Verification items for the finished model (mm, model axes). A direction names the side the tool comes from. Coordinates: 2 decimals unless noted, no trailing zeros. Order: outer loops, then holes, each group sorted by start corner. A loop starts at its lowest first (then second) coordinate and runs counter-clockwise, first axis right, second up. Notation, with made-up numbers: M 51,82 L 62,82 A17 cw 62,94 Z; hole C -3,-40 d4. An arc over 180 degrees is marked long. Answer as a JSON object with one key per item and string values. Group by question number.
(1) Cross-section at A-A (z = 15). Enter the section's corners in (x, y), plus the area to 3 significant figures.
(2) Access from +Z, -Z, +X, -X, +Y, -Y to the whole of each face (thin tool, end or side, straight path). Record for faces 5 (the face through (-12.5, 6, -1)), 6 (the face through (0, -5.5, 27)), 7 (the face through (-15.5, 5, 0)).
(3) Mould release check, pull along X, two halves, no side actions. Record for faces 1 (the face through (20, 11, -13)), 2 (the face through (-0.341, -15.496, 0.399)), 3 (the face through (16, 12.5, 0)), 4 (the face through (23.5, 11, 0)): released by +X, released by -X, zero draft, split by the parting line, or undercut.
(4) Gauge pin test, flat ends, axial feed: pin 1 Ø4 at (y, z) = (4.5, 4.5) entering from +X; pin 2 Ø6 at (x, z) = (10, -10) entering from +Y; pin 3 Ø1.5 at (y, z) = (0.5, 27.5) entering from -X; pin 4 Ø6.5 at (x, z) = (17.5, 11.5) entering from -Y. Record the tip position at first contact, or that the pin passes through.
(5) Cross-section at D-D (x = 10). Enter the section's corners in (y, z), plus the area to 3 significant figures.
(6) Cross-section at C-C (z = -19). Enter the section's corners in (x, y).
(7) Cross-section at B-B (x = -18). Enter the section's corners in (y, z), plus the area to 3 significant figures.
(8) Material ranges on line 1 (Z direction, x = -18, y = 11.95); line 2 (X direction, y = 0.25, z = -4); line 3 (Y direction, x = 0, z = 20), recorded low to high.
from build123d import *

# Parameters (mm, degrees)
SALIENTE_EXTRUIR1_DEPTH = 28.5
CROQUIS2_R              = 2
CORTAR_EXTRUIR1_DEPTH   = 5
SALIENTE_EXTRUIR2_DEPTH = 3
CROQUIS4_W              = 5
CROQUIS4_H              = 3
CROQUIS4_W_2            = 7
CROQUIS4_H_2            = 13
CORTAR_EXTRUIR3_DEPTH   = 3


with BuildPart() as part:
    # Croquis1 → Saliente-Extruir1 (new, symmetric)
    with BuildSketch(Plane.XY):
        with BuildLine():
            Line((-12.5, 0), (-12.5, 12.5))
            Line((-12.5, 12.5), (-23.5, 12.5))
            Line((-23.5, 12.5), (-23.5, 9.5))
            Line((-23.5, 9.5), (-15.5, 9.5))
            Line((-15.5, 9.5), (-15.5, 0))
            ThreePointArc((-15.5, 0), (0, -15.5), (15.5, 0))
            Line((15.5, 0), (15.5, 9.5))
            Line((15.5, 9.5), (23.5, 9.5))
            Line((23.5, 9.5), (23.5, 12.5))
            Line((23.5, 12.5), (12.5, 12.5))
            Line((12.5, 12.5), (12.5, 0))
            ThreePointArc((12.5, 0), (0, -12.5), (-12.5, 0))
        make_face()
    extrude(amount=SALIENTE_EXTRUIR1_DEPTH, both=True)

    # Croquis2 → Cortar-Extruir1 (cut)
    with BuildSketch(Plane.XZ.offset(-9.5)):
        with Locations((-18, 15)):
            Circle(CROQUIS2_R)
        with Locations((-18, -15)):
            Circle(CROQUIS2_R)
        with Locations((20, 15)):
            Circle(CROQUIS2_R)
        with Locations((20, -15)):
            Circle(CROQUIS2_R)
    extrude(amount=-CORTAR_EXTRUIR1_DEPTH, mode=Mode.SUBTRACT)

    # Croquis3 → Saliente-Extruir2 (add)
    with BuildSketch(Plane.XY.offset(28.5)):
        with BuildLine():
            Line((-15.5, 12.5), (15.5, 12.5))
            Line((15.5, 12.5), (15.5, 0))
            ThreePointArc((15.5, 0), (0, -15.5), (-15.5, 0))
            Line((-15.5, 0), (-15.5, 12.5))
        make_face()
    extrude(amount=-SALIENTE_EXTRUIR2_DEPTH)

    # Croquis4 → Cortar-Extruir3 (cut)
    with BuildSketch(Plane.XY.offset(28.5)):
        with Locations((-8.6, 0)):
            Rectangle(CROQUIS4_W, CROQUIS4_H)
        with Locations((0, 1)):
            Rectangle(CROQUIS4_W_2, CROQUIS4_H_2)
        with Locations((8.6, 0)):
            Rectangle(CROQUIS4_W, CROQUIS4_H)
    extrude(amount=-CORTAR_EXTRUIR3_DEPTH, mode=Mode.SUBTRACT)


solid = part.part
Taken from the geometry:
{
 "1": {"outline": "M -23.5,9.5 L -20,9.5 L -20,12.5 L -23.5,12.5 Z; M -16,9.5 L -15.5,9.5 L -15.5,0 A15.5 ccw 15.5,0 L 15.5,9.5 L 18,9.5 L 18,12.5 L 12.5,12.5 L 12.5,0 A12.5 cw -12.5,0 L -12.5,12.5 L -16,12.5 Z; M 22,9.5 L 23.5,9.5 L 23.5,12.5 L 22,12.5 Z", "area": "231 mm²"},
 "2": {"face 5": "-Z, +Y", "face 6": "+Z, -Z", "face 7": "+Z, -Z, -X, -Y"},
 "3": {"face 1": "undercut", "face 2": "split by the parting line", "face 3": "zero draft", "face 4": "released by +X"},
 "4": {"pin 1": "stops at x = 15.5", "pin 2": "stops at y = 12.5", "pin 3": "stops at x = -15.5", "pin 4": "stops at y = -6.1"},
 "5": {"outline": "M -11.84,-28.5 L -7.5,-28.5 L -7.5,25.5 L -1.5,25.5 L -1.5,28.5 L -11.84,28.5 Z; M 1.5,25.5 L 12.5,25.5 L 12.5,28.5 L 1.5,28.5 Z", "area": "299 mm²"},
 "6": {"outline": "M -23.5,9.5 L -15.5,9.5 L -15.5,0 A15.5 ccw 15.5,0 L 15.5,9.5 L 23.5,9.5 L 23.5,12.5 L 12.5,12.5 L 12.5,0 A12.5 cw -12.5,0 L -12.5,12.5 L -23.5,12.5 Z"},
 "7": {"outline": "M 9.5,-28.5 L 12.5,-28.5 L 12.5,-17 L 9.5,-17 Z; M 9.5,-13 L 12.5,-13 L 12.5,13 L 9.5,13 Z; M 9.5,17 L 12.5,17 L 12.5,28.5 L 9.5,28.5 Z", "area": "147 mm²"},
 "8": {"line 1": "z = -28.5 to -17, -13 to 13, 17 to 28.5", "line 2": "x = -15.5 to -12.5, 12.5 to 15.5", "line 3": "y = -15.5 to -12.5"}
}
